Geometry: final body of the model. Coordinates: model frame, mm. Face numbers are marked on the shaded views. A direction names the side the tool comes from. Give positions to 0.01 mm unless a question says otherwise; leave off trailing zeros. Write each loop counter-clockwise with the first axis right and the second up, starting at its lowest first coordinate (ties: lowest second). Pieces come first, ordered by that corner, then holes. Notation, with made-up numbers: (20, 43) - (56, 43) arc R33 cw to (56, 72) - close; hole circle Ø11 at (7, 73.25). An arc over 180 degrees is marked (long way). Return JSON: item names as keys, results as strings.
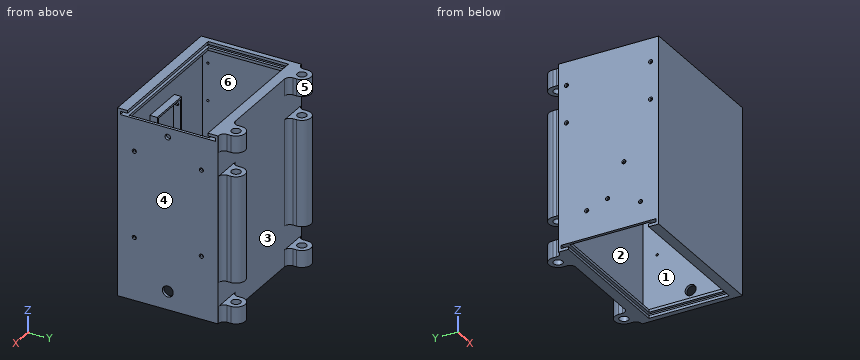
from build123d import *

# Parameters (mm, degrees)
SKETCH1_R                        = 6.35
BODY_EXTRUDE_DEPTH               = 260.35
ATTACHMENT_FILLET_R              = 7.62
BACK_DOOR_CUT_DEPTH              = 199.39
SKETCH4_3_W                      = 3.81
SKETCH4_3_H                      = 111.76
BACK_DOOR_CUT_2_DEPTH            = 195.58
FRONT_DOOR_CUT_START             = -3.81
SKETCH4_5_W                      = 4.572
SKETCH4_5_H                      = 132.08
FRONT_DOOR_CUT_DEPTH             = 340.912162509
FRONT_DOOR_CUT_2_START           = -7.62
SKETCH4_6_W                      = 3.81
SKETCH4_6_H                      = 111.76
FRONT_DOOR_CUT_2_DEPTH           = 337.102162509
SKETCH5_W                        = 203.2
SKETCH5_H                        = 33.02
STOPPER_CUT_DEPTH                = 313.443230844
SKETCH6_W                        = 195.58
SKETCH6_H                        = 132.08
HOLLOW_CUT_DEPTH                 = 243.586
SKETCH7_W                        = 3.81
SKETCH7_H                        = 10.16
INNER_RAIL_EXTRUDE_DEPTH         = 195.58
BATTERY_RAILS_EXTRUDE_DEPTH      = 10.16
BATTERY_RAIL_HOLES_CUT_REACH     = 308.701
SKETCH12_R                       = 2.54
USRP_HOLES_D                     = 3.2639
USRP_HOLES_DEPTH                 = 3.81
USRP_HOLES_CSINK_D               = 5.715
USRP_HOLES_CSINK_ANGLE           = 100
JETSON_HOLES_D                   = 3.2639
JETSON_HOLES_DEPTH               = 3.81
JETSON_HOLES_CSINK_D             = 5.715
JETSON_HOLES_CSINK_ANGLE         = 100
CUI_HOLES_D                      = 3.2639
CUI_HOLES_DEPTH                  = 3.81
CUI_HOLES_CSINK_D                = 5.715
CUI_HOLES_CSINK_ANGLE            = 100
SKETCH19_W                       = 7.62
SKETCH19_H                       = 3.81
INNER_DOOR_STOPPERS_DEPTH        = 135.89
TERMINAL_BLOCK_HOLES_D           = 3.2639
TERMINAL_BLOCK_HOLES_DEPTH       = 3.81
TERMINAL_BLOCK_HOLES_CSINK_D     = 5.715
TERMINAL_BLOCK_HOLES_CSINK_ANGLE = 100
SKETCH23_R                       = 3.81
SKETCH23_R_2                     = 7.62
MARINE_SEAL_DEPTH                = 3.81


with BuildPart() as part:
    # Sketch1 → body_extrude (new body)
    with BuildSketch(Plane.XY):
        with BuildLine():
            Line((-92.6973, 69.85), (-92.6973, 82.55))
            ThreePointArc((-92.6973, 82.55), (-79.9973, 95.25), (-67.2973, 82.55))
            Line((-67.2973, 82.55), (-67.2973, 69.85))
            Line((-67.2973, 69.85), (67.2973, 69.85))
            Line((67.2973, 69.85), (67.2973, 82.55))
            ThreePointArc((67.2973, 82.55), (79.9973, 95.25), (92.6973, 82.55))
            Line((92.6973, 82.55), (92.6973, 69.85))
            Line((92.6973, 69.85), (101.6, 69.85))
            Line((101.6, 69.85), (101.6, -69.85))
            Line((101.6, -69.85), (-101.6, -69.85))
            Line((-101.6, -69.85), (-101.6, 69.85))
            Line((-101.6, 69.85), (-92.6973, 69.85))
        make_face()
        with Locations((-79.9973, 82.55)):
            Circle(SKETCH1_R, mode=Mode.SUBTRACT)
        with Locations(Location((79.9973, 82.55, 0), (0, 0, 180))):
            Circle(SKETCH1_R, mode=Mode.SUBTRACT)
    extrude(amount=BODY_EXTRUDE_DEPTH)

    # attachment_fillet
    attachment_fillet_edges = [part.edges().sort_by_distance(p)[0] for p in [
        (-92.6973, 69.85, 130.175),
        (-67.2973, 69.85, 130.175),
        (67.2973, 69.85, 130.175),
        (92.6973, 69.85, 130.175),
    ]]
    fillet(attachment_fillet_edges, radius=ATTACHMENT_FILLET_R)

    # Sketch4 → back_door_cut (cut)
    with BuildSketch(Plane.ZY.offset(101.6)):
        Polygon((3.81, 55.88), (3.81, -55.88), (3.81, -66.04), (8.382, -66.04), (8.382, 66.04), (3.81, 66.04), align=None)
    extrude(amount=-BACK_DOOR_CUT_DEPTH, mode=Mode.SUBTRACT)

    # Sketch4<3> → back_door_cut_2 (cut)
    with BuildSketch(Plane.ZY.offset(101.6)):
        with Locations((1.905, 0)):
            Rectangle(SKETCH4_3_W, SKETCH4_3_H)
    extrude(amount=-BACK_DOOR_CUT_2_DEPTH, mode=Mode.SUBTRACT)

    # Sketch4<5> → front_door_cut (cut, through all)
    with BuildSketch(Plane.ZY.offset(101.6).offset(FRONT_DOOR_CUT_START)):
        with Locations((254.254, 0)):
            Rectangle(SKETCH4_5_W, SKETCH4_5_H)
    extrude(amount=-FRONT_DOOR_CUT_DEPTH, mode=Mode.SUBTRACT)

    # Sketch4<6> → front_door_cut_2 (cut, through all)
    with BuildSketch(Plane.ZY.offset(101.6).offset(FRONT_DOOR_CUT_2_START)):
        with Locations((258.445, 0)):
            Rectangle(SKETCH4_6_W, SKETCH4_6_H)
    extrude(amount=-FRONT_DOOR_CUT_2_DEPTH, mode=Mode.SUBTRACT)

    # Sketch5 → stopper_cut (cut, through all)
    with BuildSketch(Plane(origin=(0, 69.85, 0), x_dir=(1, 0, 0), z_dir=(0, 1, 0))):
        with Locations((0, -40.005)):
            Rectangle(SKETCH5_W, SKETCH5_H)
        with Locations((0, -220.345)):
            Rectangle(SKETCH5_W, SKETCH5_H)
    extrude(amount=STOPPER_CUT_DEPTH, mode=Mode.SUBTRACT)

    # Sketch6 → hollow_cut (cut)
    with BuildSketch(Plane(origin=(0, 0, 8.382), x_dir=(-1, 0, 0), z_dir=(0, 0, -1))):
        Rectangle(SKETCH6_W, SKETCH6_H)
    extrude(amount=-HOLLOW_CUT_DEPTH, mode=Mode.SUBTRACT)

    # Sketch7 → inner_rail_extrude (add)
    with BuildSketch(Plane.ZY.offset(97.79)):
        with Locations((10.287, -60.96)):
            Rectangle(SKETCH7_W, SKETCH7_H)
        with Locations((10.287, 60.96)):
            Rectangle(SKETCH7_W, SKETCH7_H)
        with Locations((250.063, -60.96)):
            Rectangle(SKETCH7_W, SKETCH7_H)
        with Locations((250.063, 60.96)):
            Rectangle(SKETCH7_W, SKETCH7_H)
    extrude(amount=-INNER_RAIL_EXTRUDE_DEPTH)

    # Sketch11 → battery_rails_extrude (add)
    with BuildSketch(Plane.XZ.offset(66.04)):
        Polygon((-27.051, 213.106), (27.051, 213.106), (27.051, 47.244), (27.051, 44.704), (29.591, 44.704), (29.591, 215.646), (-29.591, 215.646), (-29.591, 44.704), (-27.051, 44.704), (-27.051, 47.244), align=None)
    extrude(amount=-BATTERY_RAILS_EXTRUDE_DEPTH)

    # battery_rail_holes_cut: up to this face of the body (flat: up to its plane)
    battery_rail_holes_cut_end = Plane(part.part.faces().sort_by_distance((29.591, -60.96, 130.175))[0])
    # Sketch12 → battery_rail_holes_cut (cut, up to the picked face)
    with BuildSketch(Plane.ZY.offset(29.591), mode=Mode.PRIVATE) as battery_rail_holes_cut_sk1:
        with Locations((54.864, -60.96)):
            Circle(SKETCH12_R)
    battery_rail_holes_cut_tool1 = split(extrude(battery_rail_holes_cut_sk1.sketch, amount=-BATTERY_RAIL_HOLES_CUT_REACH, mode=Mode.PRIVATE), bisect_by=battery_rail_holes_cut_end, keep=Keep.BOTH, mode=Mode.PRIVATE)
    # Sketch12 → battery_rail_holes_cut (cut, up to the picked face)
    with BuildSketch(Plane.ZY.offset(29.591), mode=Mode.PRIVATE) as battery_rail_holes_cut_sk2:
        with Locations((130.175, -60.96)):
            Circle(SKETCH12_R)
    battery_rail_holes_cut_tool2 = split(extrude(battery_rail_holes_cut_sk2.sketch, amount=-BATTERY_RAIL_HOLES_CUT_REACH, mode=Mode.PRIVATE), bisect_by=battery_rail_holes_cut_end, keep=Keep.BOTH, mode=Mode.PRIVATE)
    # Sketch12 → battery_rail_holes_cut (cut, up to the picked face)
    with BuildSketch(Plane.ZY.offset(29.591), mode=Mode.PRIVATE) as battery_rail_holes_cut_sk3:
        with Locations((205.486, -60.96)):
            Circle(SKETCH12_R)
    battery_rail_holes_cut_tool3 = split(extrude(battery_rail_holes_cut_sk3.sketch, amount=-BATTERY_RAIL_HOLES_CUT_REACH, mode=Mode.PRIVATE), bisect_by=battery_rail_holes_cut_end, keep=Keep.BOTH, mode=Mode.PRIVATE)
    add(battery_rail_holes_cut_tool1.solids().sort_by(Axis((-29.591, -60.96, 54.864), (1, 0, 0)))[0], mode=Mode.SUBTRACT)
    add(battery_rail_holes_cut_tool2.solids().sort_by(Axis((-29.591, -60.96, 130.175), (1, 0, 0)))[0], mode=Mode.SUBTRACT)
    add(battery_rail_holes_cut_tool3.solids().sort_by(Axis((-29.591, -60.96, 205.486), (1, 0, 0)))[0], mode=Mode.SUBTRACT)

    # usrp_holes
    with Locations(Plane(origin=(101.6, 0, 0), x_dir=(0, 0, -1), z_dir=(1, 0, 0))):
        with Locations((-87.1982, 46.609), (-206.5528, 46.609), (-206.5528, -46.609), (-87.1982, -46.609)):
            CounterSinkHole(USRP_HOLES_D / 2, USRP_HOLES_CSINK_D / 2, depth=USRP_HOLES_DEPTH, counter_sink_angle=USRP_HOLES_CSINK_ANGLE)

    # jetson_holes
    with Locations(Plane.ZY.offset(101.6)):
        with Locations((175.9712, -58.4454), (175.9712, 58.4454), (227.8888, 58.4454), (227.8888, -58.4454)):
            CounterSinkHole(JETSON_HOLES_D / 2, JETSON_HOLES_CSINK_D / 2, depth=JETSON_HOLES_DEPTH, counter_sink_angle=JETSON_HOLES_CSINK_ANGLE)

    # cui_holes
    with Locations(Plane.ZY.offset(101.6)):
        with Locations((99.822, -21.336), (38.1, -44.45)):
            CounterSinkHole(CUI_HOLES_D / 2, CUI_HOLES_CSINK_D / 2, depth=CUI_HOLES_DEPTH, counter_sink_angle=CUI_HOLES_CSINK_ANGLE)

    # Sketch19 → inner_door_stoppers (add)
    with BuildSketch(Plane.XZ.offset(69.85)):
        with Locations((97.79, 10.287)):
            Rectangle(SKETCH19_W, SKETCH19_H)
        with Locations((-97.79, 250.063)):
            Rectangle(SKETCH19_W, SKETCH19_H)
    extrude(amount=-INNER_DOOR_STOPPERS_DEPTH)

    # terminal_block_holes
    with Locations(Plane.ZY.offset(101.6)):
        with Locations((55.1815, 1.27), (46.4185, 30.353)):
            CounterSinkHole(TERMINAL_BLOCK_HOLES_D / 2, TERMINAL_BLOCK_HOLES_CSINK_D / 2, depth=TERMINAL_BLOCK_HOLES_DEPTH, counter_sink_angle=TERMINAL_BLOCK_HOLES_CSINK_ANGLE)

    # Sketch23 → marine_seal (cut)
    with BuildSketch(Plane(origin=(101.6, 0, 0), x_dir=(0, 0, -1), z_dir=(1, 0, 0))):
        with Locations(Location((-239.268, 0, 0), (0, 0, 90))):
            Circle(SKETCH23_R)
        with Locations(Location((-25.4, 0, 0), (0, 0, 90))):
            Circle(SKETCH23_R_2)
    extrude(amount=-MARINE_SEAL_DEPTH, mode=Mode.SUBTRACT)


solid = part.part
Q1. Pin query (flat end, axial travel): P1, Ø3, axis at y = 76, z = 187.5, coming from the +X side; P2, Ø3, axis at y = -44.45, z = 38.1, coming from the -X side; P3, Ø3.5, axis at y = 2, z = 254, coming from the +X side; P4, Ø1.5, axis at x = -58.5, y = 72.5, coming from the +Z side. Return the tip coordinate at first contact, or that it passes through.
Answer key:
{"P1": "stops at x = 93.3", "P2": "stops at x = 97.79", "P3": "stops at x = -97.79", "P4": "passes through"}
Q2. Section query C-C, the plane y = 13.5. Return the cut outline in (x, z).
Answer key:
{"outline": "(-101.6, 8.38) - (-97.79, 8.38) - (-97.79, 248.16) - (-93.98, 248.16) - (-93.98, 251.97) - (-97.79, 251.97) - (-97.79, 256.54) - (-93.98, 256.54) - (-93.98, 260.35) - (-101.6, 260.35) - close; (93.98, 0) - (101.6, 0) - (101.6, 251.97) - (97.79, 251.97) - (97.79, 12.19) - (93.98, 12.19) - (93.98, 8.38) - (97.79, 8.38) - (97.79, 3.81) - (93.98, 3.81) - close"}
Q3. Material intervals for probe 1 along Z at (x, y) = (83.5, 70.5) (3 decimals); probe 2 along Z at (x, y) = (-61.5, 58); probe 3 along X at (y, z) = (-62.5, 128), sorted ascending. Write a range as [from, to].
Answer key:
{"probe 1": "z = [0, 23.495], [56.515, 203.835], [236.855, 260.35]", "probe 2": "z = [0, 3.81], [8.38, 12.19], [248.16, 251.97], [256.54, 260.35]", "probe 3": "x = [-101.6, -97.79], [-29.59, -27.05], [27.05, 29.59], [97.79, 101.6]"}
Q4. Section query A-A, the plane z = 149. Count the separate pieces of the cut face and the enclosed holes in it, plus the area to 3 significant figures.
Answer key:
{"separate pieces": "1", "enclosed holes": "3", "area": "3,550 mm^2"}
Q5. Mould query, pull axis Y, two halves, no side actions, for the marked faces 1, 2, 3 and 4. Classes: pulls with the +Y half, pulls with the -Y half, needs draft (parallel to the pull), parting line crosses it, or undercut.
Answer key:
{"face 1": "undercut", "face 2": "undercut", "face 3": "pulls with the +Y half", "face 4": "needs draft"}
Q6. Set-up query: the marked faces 5 and 6. Return all of +Z, -Z, +X, -X, +Y, -Y with unobstructed straight access to the full face (end or side cutting, diameter ignored); none if empty.
Answer key:
{"face 5": "+Z, -Z, +Y", "face 6": "none"}
